Could you check a few things on this drawing? It's one solid part, dimensions in mm from its lowest x, y, z. Coordinates: 2 decimals unless noted, no trailing zeros. Write each loop counter-clockwise with the first axis right and the second up, starting at its lowest first coordinate (ties: lowest second). Pieces come first, ordered by that corner, then holes.
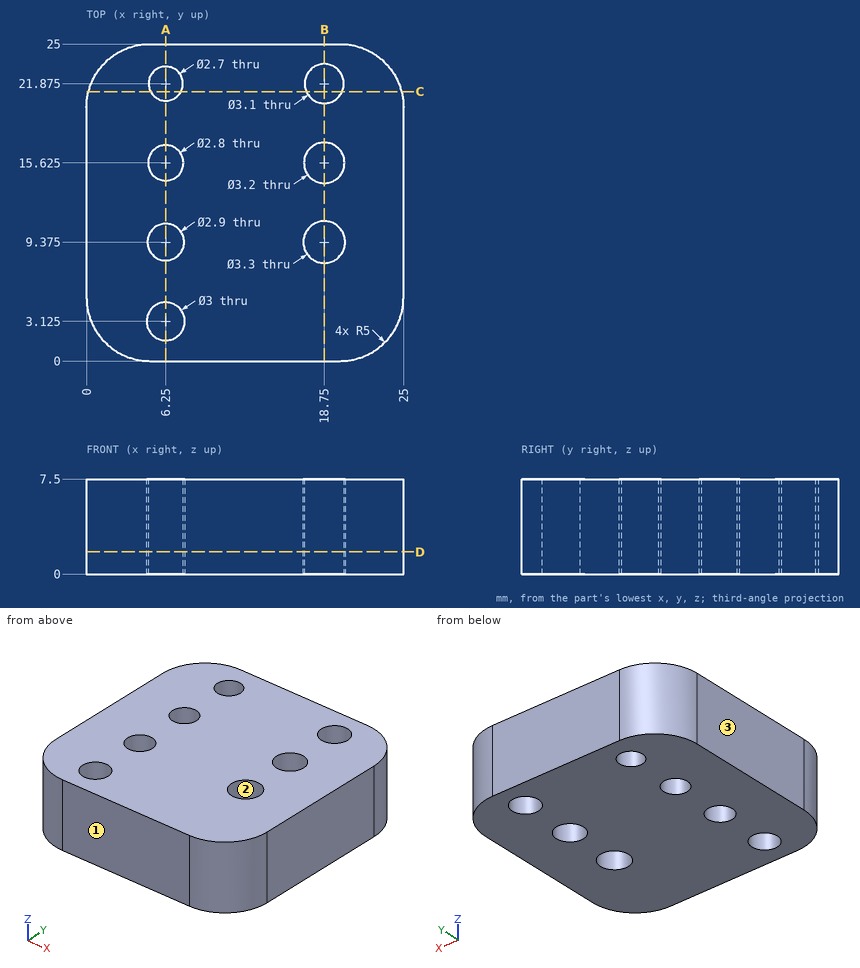
1) Imagine slicing it at C-C on y = 21.25. Please give me the cut outline in (x, z).
Values follow:
outline: (0.16, 0) - (5.05, 0) - (5.05, 7.5) - (0.16, 7.5) - close; (7.45, 0) - (17.33, 0) - (17.33, 7.5) - (7.45, 7.5) - close; (20.17, 0) - (24.84, 0) - (24.84, 7.5) - (20.17, 7.5) - close
2) Imagine slicing it at D-D on z = 1.75. Please give me the cut outline in (x, y) (3 decimals), then the cut area to 3 significant figures.
Values follow:
outline: (0, 5) arc R5 ccw to (5, 0) - (20, 0) arc R5 ccw to (25, 5) - (25, 20) arc R5 ccw to (20, 25) - (5, 25) arc R5 ccw to (0, 20) - close; hole circle Ø3 at (6.25, 3.125); hole circle Ø2.9 at (6.25, 9.375); hole circle Ø2.8 at (6.25, 15.625); hole circle Ø2.7 at (6.25, 21.875); hole circle Ø3.3 at (18.75, 9.375); hole circle Ø3.2 at (18.75, 15.625); hole circle Ø3.1 at (18.75, 21.875)
area: 554 mm2
3) Imagine slicing it at B-B on x = 18.75. Please give me the cut outline in (y, z) (3 decimals), then the cut area to 4 significant figures.
Values follow:
outline: (0, 0) - (7.725, 0) - (7.725, 7.5) - (0, 7.5) - close; (11.025, 0) - (14.025, 0) - (14.025, 7.5) - (11.025, 7.5) - close; (17.225, 0) - (20.325, 0) - (20.325, 7.5) - (17.225, 7.5) - close; (23.425, 0) - (25, 0) - (25, 7.5) - (23.425, 7.5) - close
area: 115.5 mm2
4) Will this pin go through, and if not, where does the flat tip stop? pin 1 (1.7 mm diameter, centred on x = 6.25, y = 15.625, fed in from +Z).
Values follow:
pin 1: passes through
5) We'd pull the mould along X, two halves only. Please class the marked faces 1, 2 and 3: pulls with the +X half, pulls with the -X half, needs draft (parallel to the pull), parting line crosses it, or undercut.
Values follow:
face 1: needs draft
face 2: undercut
face 3: pulls with the -X half
6) I need wall thicknesses on probe 1 along Y at (x, z) = (6.25, 4.25) (3 decimals); probe 2 along Y at (x, z) = (18.75, 6) (3 decimals); probe 3 along X at (y, z) = (21.25, 3.25). Which ranges of each line are inside material? Lowest first, please.
Values follow:
probe 1: y = 0 to 1.625, 4.625 to 7.925, 10.825 to 14.225, 17.025 to 20.525, 23.225 to 25
probe 2: y = 0 to 7.725, 11.025 to 14.025, 17.225 to 20.325, 23.425 to 25
probe 3: x = 0.16 to 5.05, 7.45 to 17.33, 20.17 to 24.84
7) Imagine slicing it at A-A on x = 6.25. Please give me the cut outline in (y, z) (3 decimals), then the cut area to 3 significant figures.
Values follow:
outline: (0, 0) - (1.625, 0) - (1.625, 7.5) - (0, 7.5) - close; (4.625, 0) - (7.925, 0) - (7.925, 7.5) - (4.625, 7.5) - close; (10.825, 0) - (14.225, 0) - (14.225, 7.5) - (10.825, 7.5) - close; (17.025, 0) - (20.525, 0) - (20.525, 7.5) - (17.025, 7.5) - close; (23.225, 0) - (25, 0) - (25, 7.5) - (23.225, 7.5) - close
area: 102 mm2
